Could you check a few things on this model? Use its own coordinates, in mm. A direction names the side the tool comes from. Round coordinates to 2 decimals unless told otherwise and drop trailing zeros. Loops run counter-clockwise (first coordinate to the right, second up) from the corner with the lowest first, then second, coordinate; pieces in that order, holes last. Notation, with made-up numbers: (60, -13.5) -> (110, -13.5) arc R25 ccw to (110, 25.5) -> close; hole circle Ø9 at (77, 58.25). An arc over 180 degrees is marked (long way). Write each question's results on one line, items separated by ' | '.
from build123d import *

# Parameters (mm, degrees)
F0_W       = 52.5342468172
F0_H       = 49.9637834728
F1_DEPTH   = 48.514
F2_W       = 48.514
F2_H       = 24.9818917364
F3_DEPTH   = 46.99
F4_W       = 48.514
F4_H       = 24.9818917364
F5_DEPTH   = 49.53
F6_W       = 48.514
F6_H       = 49.53
F7_DEPTH   = 45.72
F8_W       = 48.514
F8_H       = 46.99
F9_DEPTH   = 45.974
F10_W      = 48.514
F10_H      = 46.99
F11_DEPTH  = 137.922
F12_DEPTH  = 140.208
F13_W      = 48.514
F13_H      = 208.8778917364
F14_DEPTH  = 153.162
F15_W      = 48.514
F15_H      = 208.8778917364
F12_FACE_W = 48.514
F12_FACE_H = 210.9098917364
F16_DEPTH  = 25.4
F17_DEPTH  = 189.484


with BuildPart() as f1:
    # F0 (on Right) → F1 (new body)
    with BuildSketch(Plane.YZ):
        with Locations((-53.4399999306, 24.9818917364)):
            Rectangle(F0_W, F0_H)
    extrude(amount=F1_DEPTH)

    # F2 (on face) → F3 (join)
    with BuildSketch(Plane.XZ.offset(79.7071233392)):
        with Locations((24.257, 12.4909458682)):
            Rectangle(F2_W, F2_H)
    extrude(amount=F3_DEPTH)

    # F4 (on face) → F5 (join)
    with BuildSketch(Plane(origin=(0, -27.1728765219, 0), x_dir=(-1, 0, 0), z_dir=(0, 1, 0))):
        with Locations((-24.257, 12.4909458682)):
            Rectangle(F4_W, F4_H)
    extrude(amount=F5_DEPTH)

    # F6 (on face) → F7 (join)
    with BuildSketch(Plane.XY.offset(24.9818917364)):
        with Locations((24.257, -2.4078765219)):
            Rectangle(F6_W, F6_H)
    extrude(amount=F7_DEPTH)

    # F8 (on face) → F9 (join)
    with BuildSketch(Plane.XY.offset(24.9818917364)):
        with Locations((24.257, -103.2021233392)):
            Rectangle(F8_W, F8_H)
    extrude(amount=F9_DEPTH)

    # F10 (on face) → F11 (join)
    with BuildSketch(Plane.XY.offset(70.9558917364)):
        with Locations((24.257, -103.2021233392)):
            Rectangle(F10_W, F10_H)
    extrude(amount=F11_DEPTH)

    # F12 (add): a face of the model
    f12_faces = [f1.faces().sort_by_distance(p)[0] for p in [
        (24.257, -2.4078765219, 70.7018917364),
    ]]
    extrude(f12_faces, amount=F12_DEPTH)

    # F13 (on face) → F14 (join)
    with BuildSketch(Plane.XZ.offset(126.6971233392)):
        with Locations((24.257, 104.4389458682)):
            Rectangle(F13_W, F13_H)
    extrude(amount=F14_DEPTH)

    # F15 (on face) + F12_face (on face) → F16 (join)
    with BuildSketch(Plane.XZ.offset(279.8591233392)):
        with Locations((24.257, 104.4389458682)):
            Rectangle(F15_W, F15_H)
    with BuildSketch(Plane(origin=(24.257, 22.3571234781, 105.4549458682), x_dir=(-1, 0, 0), z_dir=(0, 1, 0))):
        Rectangle(F12_FACE_W, F12_FACE_H)
    extrude(amount=F16_DEPTH, dir=(0, -1, 0))

    # F17 (add): a face of the model
    f17_faces = [f1.faces().sort_by_distance(p)[0] for p in [
        (24.257, 22.3571234781, 105.4549458682),
    ]]
    extrude(f17_faces, amount=F17_DEPTH)


solid = f1.part
1) For faces 1 (the flat face through (24, -191, 208.878)), 2 (the flat face through (24, -79.707, 128)), 3 (the flat face through (24, 91, 210.91)), which set-ups out of +Z, -Z, +X, -X, +Y, -Y let a thin tool reach every point of the face, with its end or its side?
Model answer:
face 1: +Z, +X, -X, -Y | face 2: +Z, +X, -X | face 3: +Z, +X, -X, +Y, -Y
2) I need wall thicknesses on line 1 (Y direction, x = 14.5, z = 98.5); line 2 (Z direction, x = 13, y = -273.5); line 3 (Z direction, x = 9.5, y = -44). Which ranges of each line are inside material? Lowest first, please.
Model answer:
line 1: y = -305.26 to -79.71, -27.17 to 211.84 | line 2: z = 0 to 208.88 | line 3: z = 0 to 49.96
3) I want a section at C-C, the plane y = -57. Write out the boundary of the cut face in (x, z), plus the area to 3 significant figures.
Model answer:
outline: (0, 0) -> (48.51, 0) -> (48.51, 49.96) -> (0, 49.96) -> close | area: 2,420 mm2
4) I want a section at A-A, the plane z = 174.5. Write out the boundary of the cut face in (x, y).
Model answer:
outline: (0, -305.26) -> (48.51, -305.26) -> (48.51, -79.71) -> (0, -79.71) -> close; (0, -27.17) -> (48.51, -27.17) -> (48.51, 211.84) -> (0, 211.84) -> close
5) I'm going to push flat-ended pins straight in: pin 1 (12 mm diameter, centred on x = 23.5, y = -138, fed in from +Z); pin 2 (14.5 mm diameter, centred on x = 21, y = -46.5, fed in from +Z). Where does each tip first touch, or does it pass through?
Model answer:
pin 1: stops at z = 208.88 | pin 2: stops at z = 49.96
6) I want a section at B-B, the plane x = 12.5. Write out the boundary of the cut face in (y, z), plus the area to 3 significant figures.
Model answer:
outline: (-305.26, 0) -> (211.84, 0) -> (211.84, 210.91) -> (-27.17, 210.91) -> (-27.17, 49.96) -> (-79.71, 49.96) -> (-79.71, 208.88) -> (-305.26, 208.88) -> close | area: 100,000 mm2
